```python
from build123d import *

# Parameters (mm, degrees)
SKETCH1_R                     = 17.5
SKETCH1_R_2                   = 13.5
SKETCH2_R                     = 17.5
PIPE_TAP_DRILL_FOR_3_4_TAP1_D = 23.0124


with BuildPart() as part:
    # Sweep1: sweep along a curve in space
    with BuildLine() as sweep1_path:
        Line((0, 0, 0), (0, 0, -19))
    # Sketch1 → Sweep1 (sweep)
    with BuildSketch(Plane.XY):
        Circle(SKETCH1_R)
        Circle(SKETCH1_R_2, mode=Mode.SUBTRACT)
    sweep(path=sweep1_path.line)

    # Sweep2: sweep along a curve in space
    with BuildLine() as sweep2_path:
        Line((0, 0, -19), (0, 0, -38))
    # Sketch2 → Sweep2 (sweep)
    with BuildSketch(Plane(origin=(0, 0, -19), x_dir=(-1, 0, 0), z_dir=(0, 0, -1))):
        Circle(SKETCH2_R)
    sweep(path=sweep2_path.line)

    # Pipe Tap Drill for 3/4 Tap1 (through all)
    with Locations(Plane(origin=(0, 0, -38), x_dir=(-1, 0, 0), z_dir=(0, 0, -1))):
        with Locations((0, 0)):
            Hole(PIPE_TAP_DRILL_FOR_3_4_TAP1_D / 2)


solid = part.part
```
Geometry check sheet. Reference: the model listing, model coordinates, mm. A direction names the side the tool comes from. Coordinates: 2 decimals unless noted, no trailing zeros. Loops run counter-clockwise (first coordinate to the right, second up) from the corner with the lowest first, then second, coordinate; pieces in that order, holes last. Notation, with made-up numbers: (13, 8) - (37, 8) arc R28 ccw to (37, 33) - close; hole circle Ø8 at (-39.5, 2). An arc over 180 degrees is marked (long way). One line per item, written item: value. Start each with the question number.
(1) Depth check by flat-ended pin: P1, Ø2, axis at x = -6.5, z = -31.5, coming from the +Y side; P2, Ø18.5, axis at x = 0, y = 0, coming from the +Z side; P3, Ø1, axis at x = 2, z = -27.5, coming from the +Y side; P4, Ø6, axis at y = -7.5, z = -22, coming from the -X side. Enter the tip coordinate at first touch or a pass-through.
(2) Material ranges on line 1 (Y direction, x = 0, z = -24.25); line 2 (Y direction, x = 0, z = -9.5); line 3 (X direction, y = -0.5, z = -6.5), recorded low to high. Write a range as [from, to].
(3) Cross-section at C-C on z = -18. Enter the section's corners in (x, y).
(4) Tool access check on faces 1 (the cylindrical face through (-2.93, 13.18, -9.63)), 2 (the flat face through (-4, -11, -38)). Record the directions out of +Z, -Z, +X, -X, +Y, -Y that give a thin tool (end or side, any length) a straight path to the whole face; none if there is none.
(5) Cross-section at A-A on x = 0. Enter the section's corners in (y, z).
(6) Cross-section at D-D on x = -14.5. Enter the section's corners in (y, z).
(7) Mould release check, pull along X, two halves, no side actions. Record for faces 3 (the cylindrical face through (-1.154, 17.462, -19.266)), 4 (the flat face through (-10, 6, -19)), 5 (the flat face through (9, -10.3, 0)): released by +X, released by -X, zero draft, split by the parting line, or undercut.
Results below:
1. P1: stops at y = 16.61
1. P2: passes through
1. P3: stops at y = 17.44
1. P4: stops at x = -16.91
2. line 1: y = [-17.5, -11.51], [11.51, 17.5]
2. line 2: y = [-17.5, -13.5], [13.5, 17.5]
2. line 3: x = [-17.49, -13.49], [13.49, 17.49]
3. outline: circle Ø35 at (0, 0); hole circle Ø27 at (0, 0)
4. face 1: +Z
4. face 2: -Z, +X, -X, +Y, -Y
5. outline: (-17.5, -38) - (-11.51, -38) - (-11.51, -19) - (-13.5, -19) - (-13.5, 0) - (-17.5, 0) - close; (11.51, -38) - (17.5, -38) - (17.5, 0) - (13.5, 0) - (13.5, -19) - (11.51, -19) - close
6. outline: (-9.8, -38) - (9.8, -38) - (9.8, 0) - (-9.8, 0) - close
7. face 3: split by the parting line
7. face 4: undercut
7. face 5: zero draft
